Geometry: final body of the model. Coordinates: model frame, mm. Face numbers are marked on the shaded views. Coordinates: 2 decimals unless noted, no trailing zeros. Order: outer loops, then holes, each group sorted by start corner. A loop starts at its lowest first (then second) coordinate and runs counter-clockwise, first axis right, second up. Notation, with made-up numbers: (-1.5, 22.25) - (26.5, 22.25) arc R27 cw to (26.5, 60.25) - close; hole circle Ø8 at (1, 75). An arc over 180 degrees is marked (long way). Use a Markdown table: item, result. Add a question column.
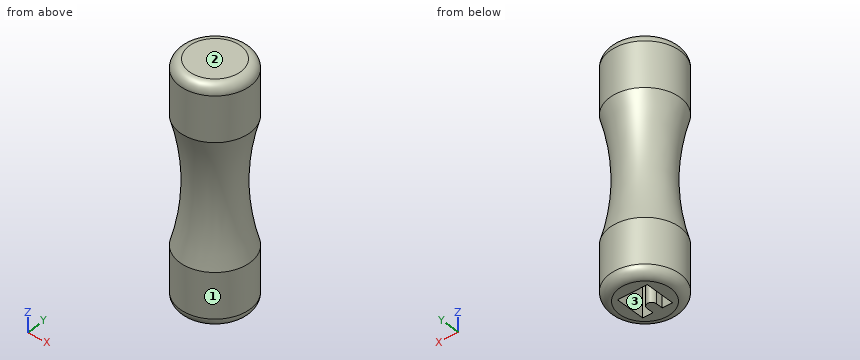
```python
from build123d import *

# Parameters (mm, degrees)
F0_R     = 7.5
F1_DEPTH = 50
F3_DEPTH = 25
F6_R     = 2


with BuildPart() as f1:
    # F0 (on Top) → F1 (new body)
    with BuildSketch(Plane.XY):
        Circle(F0_R)
    extrude(amount=F1_DEPTH)

    # F2 (on Top) → F3 (cut)
    with BuildSketch(Plane.XY):
        with BuildLine():
            Line((3.2, -3.2), (3.2, 3.2))
            Line((3.2, 3.2), (-3.2, 3.2))
            Line((-3.2, 3.2), (-3.2, -3.2))
            Line((-3.2, -3.2), (-1, -3.2))
            Line((-1, -3.2), (-1, -1.7))
            ThreePointArc((-1, -1.7), (0, -0.7), (1, -1.7))
            Line((1, -1.7), (1, -3.2))
            Line((1, -3.2), (3.2, -3.2))
        make_face()
    extrude(amount=F3_DEPTH, mode=Mode.SUBTRACT)

    # F4 (on Front) → F5 (revolve, cut)
    with BuildSketch(Plane.XZ):
        with BuildLine():
            ThreePointArc((-8, 10), (-5.596052, 25), (-8, 40))
            Line((-8, 40), (-13, 40))
            Line((-13, 40), (-13, 10))
            Line((-13, 10), (-8, 10))
        make_face()
    revolve(axis=Axis((0, 0, 50), (0, 0, 1)), mode=Mode.SUBTRACT)

    # F6
    f6_edges = [f1.edges().sort_by_distance(p)[0] for p in [
        (-7.5, 0, 50),
        (-7.5, 0, 0),
    ]]
    fillet(f6_edges, radius=F6_R)


solid = f1.part
```
1) Section query D-D (z = 37.5). Return the cut outline in (x, y), and give its area (3 significant figures).
2) Section query A-A (x = 0). Return the cut outline in (y, z).
3) Draft query along X for the marked faces 1, 2 and 3. Return one class per face: released by +X, released by -X, zero draft, split by the parting line, or undercut.
4) First-contact query: pin 1 (2 mm diameter, centred on x = -4.5, y = -5.5, fed in from +Z); pin 2 (1 mm diameter, centred on x = 3.5, z = 14.5, fed in from -Y); pin 3 (2 mm diameter, centred on y = 4.5, z = 36.5, fed in from -X). Flat tips, straight axial feed; report the tip coordinate or a pass-through.
5) Section query C-C (z = 30). Return the cut outline in (x, y), and give its area (3 significant figures).
6) Line query: line 1 (X direction, y = -1, z = 20); line 2 (Y direction, x = -3, z = 15); line 3 (Y direction, x = -2.5, z = 5). Output: solid intervals per line, ascending. Write a range as from..to.
7) Section query B-B (y = 0). Return the cut outline in (x, z).
From the geometry:
| question | item | result |
|---|---|---|
| 1 | outline | circle Ø14.5 at (0, 0) |
| 1 | area | 165 mm^2 |
| 2 | outline | (-7.5, 2) arc R2 ccw to (-5.5, 0) - (-0.7, 0) - (-0.7, 25) - (3.2, 25) - (3.2, 0) - (5.5, 0) arc R2 ccw to (7.5, 2) - (7.5, 11.62) arc R48 cw to (7.5, 38.38) - (7.5, 48) arc R2 ccw to (5.5, 50) - (-5.5, 50) arc R2 ccw to (-7.5, 48) - (-7.5, 38.38) arc R48 cw to (-7.5, 11.62) - close |
| 3 | face 1 | split by the parting line |
| 3 | face 2 | zero draft |
| 3 | face 3 | undercut |
| 4 | pin 1 | stops at z = 49.91 |
| 4 | pin 2 | stops at y = -6.09 |
| 4 | pin 3 | stops at x = -6.12 |
| 5 | outline | circle Ø11.71 at (0, 0) |
| 5 | area | 108 mm^2 |
| 6 | line 1 | x = -5.77..-3.2, -0.71..0.71, 3.2..5.77 |
| 6 | line 2 | y = -5.93..-3.2, 3.2..5.93 |
| 6 | line 3 | y = -7.07..-3.2, 3.2..7.07 |
| 7 | outline | (-7.5, 2) arc R2 ccw to (-5.5, 0) - (-3.2, 0) - (-3.2, 25) - (3.2, 25) - (3.2, 0) - (5.5, 0) arc R2 ccw to (7.5, 2) - (7.5, 11.62) arc R48 cw to (7.5, 38.38) - (7.5, 48) arc R2 ccw to (5.5, 50) - (-5.5, 50) arc R2 ccw to (-7.5, 48) - (-7.5, 38.38) arc R48 cw to (-7.5, 11.62) - close |
